from build123d import *

# Parameters (mm, degrees)
SKETCH4_R           = 5
BOSS_EXTRUDE1_DEPTH = 5
SKETCH7_R           = 1.5
BOSS_EXTRUDE2_DEPTH = 10


with BuildPart() as part:
    # Sketch4 → Boss-Extrude1 (new body)
    with BuildSketch(Plane(origin=(0, 0, 0), x_dir=(1, 0, 0), z_dir=(0, 1, 0))):
        with BuildLine():
            Line((0.951056516, 2.927050983), (20.386221797, 62.74233921))
            ThreePointArc((20.386221797, 62.74233921), (20.629049199, 64.42488908), (20.294107239, 66.091548341))
            ThreePointArc((20.294107239, 66.091548341), (0, 80), (-20.294107239, 66.091548341))
            ThreePointArc((-20.294107239, 66.091548341), (-20.629049199, 64.42488908), (-20.386221797, 62.74233921))
            Line((-20.386221797, 62.74233921), (-0.951056516, 2.927050983))
            ThreePointArc((-0.951056516, 2.927050983), (0, 2.236067977), (0.951056516, 2.927050983))
        make_face()
        with Locations((0, 71.439)):
            Circle(SKETCH4_R, mode=Mode.SUBTRACT)
    extrude(amount=BOSS_EXTRUDE1_DEPTH)

    # Sketch7 → Boss-Extrude2 (add)
    with BuildSketch(Plane(origin=(0, 5, 0), x_dir=(1, 0, 0), z_dir=(0, 1, 0))):
        with Locations((0, 62.999)):
            Circle(SKETCH7_R)
    extrude(amount=BOSS_EXTRUDE2_DEPTH)


solid = part.part
The listing builds one solid part. Answer for the finished solid, in the listing's coordinates (mm). A direction names the side the tool comes from. Coordinates: 2 decimals unless noted, no trailing zeros. Order: outer loops, then holes, each group sorted by start corner. A loop starts at its lowest first (then second) coordinate and runs counter-clockwise, first axis right, second up.
Q1. A cutting plane is placed at A-A, the plane x = 0. Write down the section's boundary in (y, z).
Q2. Consider line 1 (Z direction, x = 0, y = 1.85); line 2 (Y direction, x = -12, z = -44); line 3 (Z direction, x = 0.5, y = 4.25). Determine where each line is inside the solid, lowest interval first.
Q3. A cutting plane is placed at B-B, the plane y = 1.5. Write down the section's boundary in (x, z), and give its area (3 significant figures).
Q4. For a pull along X with two mould halves and no side action, classify faces 1 (the face through (0, 0, -50)), 2 (the face through (0, 2, -80)), 3 (the face through (-1.084, 2.465, -66.558)) as pulls with the +X half, pulls with the -X half, needs draft (parallel to the pull), parting line crosses it, or undercut.
Q5. Given P1, Ø1.5, axis at x = -3.5, z = -67.5, coming from the +Y side, flat-ended and moving along its own axis, determine where the tip first touches the part or whether it passes through.
Q6. A cutting plane is placed at D-D, the plane y = 13.5. Write down the section's boundary in (x, z).
Q7. A cutting plane is placed at C-C, the plane z = -33.5. Write down the section's boundary in (x, y), and give its area (3 significant figures).
Q8. Which of the six approach directions +Z, -Z, +X, -X, +Y, -Y give full straight-line access (tool end or side, diameter ignored) to faces 4 (the face through (-0.325, 9.93, -61.535)), 5 (the face through (0, 15, -63))?
Answers follow:
1. outline: (0, -80) - (5, -80) - (5, -76.44) - (0, -76.44) - close; (0, -66.44) - (5, -66.44) - (5, -64.5) - (15, -64.5) - (15, -61.5) - (5, -61.5) - (5, -2.24) - (0, -2.24) - close
2. line 1: z = -80 to -76.44, -66.44 to -2.24
2. line 2: y = 0 to 5
2. line 3: z = -79.99 to -76.41, -66.46 to -2.37
3. outline: (-20.39, -62.74) arc R5 ccw to (-20.29, -66.09) arc R21.76 ccw to (20.29, -66.09) arc R5 ccw to (20.39, -62.74) - (0.95, -2.93) arc R1 ccw to (-0.95, -2.93) - close; hole circle Ø10 at (0, -71.44)
3. area: 1,750 mm2
4. face 1: needs draft
4. face 2: parting line crosses it
4. face 3: undercut
5. P1: stops at y = 5
6. outline: circle Ø3 at (0, -63)
7. outline: (-10.88, 0) - (10.88, 0) - (10.88, 5) - (-10.88, 5) - close
7. area: 109 mm2
8. face 4: +Y
8. face 5: +Z, -Z, +X, -X, +Y
